Verification items for the finished model (mm, model axes). Round coordinates to 2 decimals unless told otherwise and drop trailing zeros. One line per question, with ' | ' between items.
from build123d import *

# Parameters (mm, degrees)
ESQUISSE1_R                  = 25
BOSS_EXTRU_1_DEPTH           = 18
CONG_1_R                     = 25
R_P_TITION_CIRCULAIRE1_COUNT = 3


with BuildPart() as part:
    # Esquisse1 → Boss.-Extru.1 (new body)
    with BuildSketch(Plane.XY):
        Circle(ESQUISSE1_R)
    extrude(amount=BOSS_EXTRU_1_DEPTH)

    # Congé1
    # the kernel refuses this fillet: 25 mm, written as the material it takes off along each edge
    with BuildSketch(Plane(origin=(0, 0, 18), x_dir=(1, 0, 0), z_dir=(0, -1, 0))) as cong_1_piece_1:
        with BuildLine():
            CenterArc((1, -25), CONG_1_R, 16.260204708, 73.739795292)
            Line((1, 0), (1, 0.5))
            Line((1, 0.5), (25, 0.5))
            Line((25, 0.5), (25.5, 0))
            ThreePointArc((25.5, 0), (25.5, -9), (25.48, -17.86))
            Line((25.48, -17.86), (25, -18))
        make_face()
    revolve(axis=Axis((0, 0, 18), (0, 0, 1)), mode=Mode.SUBTRACT)

    # Esquisse3 → Enlèvement de matière-Révolution1 (revolve, cut)
    with BuildSketch(Plane(origin=(0, 0, 0), x_dir=(1, 0, 0), z_dir=(0, 1, 0))):
        Polygon((16.821135137, 2.685962281), (3.656768508, -9.5900082), (5.123064982, -11.162418658), (18.287431611, 1.113551823), align=None)
    enl_vement_de_mati_re_r_volution1 = revolve(axis=Axis((0, 0, 13), (0.7313537016191742, 0, -0.6819983600624946)), mode=Mode.SUBTRACT)

    # Répétition circulaire1: Enlèvement de matière-Révolution1 ×3 about axis
    r_p_tition_circulaire1_axis = Axis((0, 0, 0), (0, 0, 1))
    for i in range(1, R_P_TITION_CIRCULAIRE1_COUNT):
        add(enl_vement_de_mati_re_r_volution1.rotate(r_p_tition_circulaire1_axis, i * 360 / R_P_TITION_CIRCULAIRE1_COUNT), mode=Mode.SUBTRACT)


solid = part.part
1. Section check A-A, the plane z = 9.75. Count the separate pieces of the cut face and the enclosed holes in it, then the cut area to 3 significant figures.
Results:
separate pieces: 1 | enclosed holes: 3 | area: 1,170 mm2
2. Thickness scan on line 1 (Z direction, x = 0, y = -3.5); line 2 (X direction, y = 9, z = 2.5); line 3 (Y direction, x = 6.5, z = 8). Record the ranges inside material, lowest first.
Results:
line 1: z = 0 to 8.47, 8.92 to 17.87 | line 2: x = -22.38 to -7.66, -3.2 to 22.38 | line 3: y = -19.97 to -2, 2 to 19.97
3. Mould release check, pull along Z, two halves, no side actions. Record for faces 1 (the face through (-5.46, -8.16, 6.67)), 2 (the face through (0, 0, 0)), 3 (the face through (0, 0, 18)): pulls with the +Z half, pulls with the -Z half, needs draft (parallel to the pull), parting line crosses it, or undercut.
Results:
face 1: undercut | face 2: pulls with the -Z half | face 3: pulls with the +Z half
4. Go/stop test with flat-tipped pins: P1, Ø1.5, axis at y = 8.5, z = 6, coming from the -X side; P2, Ø10, axis at x = -12.5, z = 13.5, coming from the +Y side; P3, Ø1.5, axis at x = -15.5, z = 2, coming from the -Y side; P4, Ø2, axis at x = 18, z = 13.5, coming from the +Y side. Record where each tip stops, or that it passes through.
Results:
P1: stops at x = -21.24 | P2: stops at y = 17.4 | P3: stops at y = -19.44 | P4: passes through
